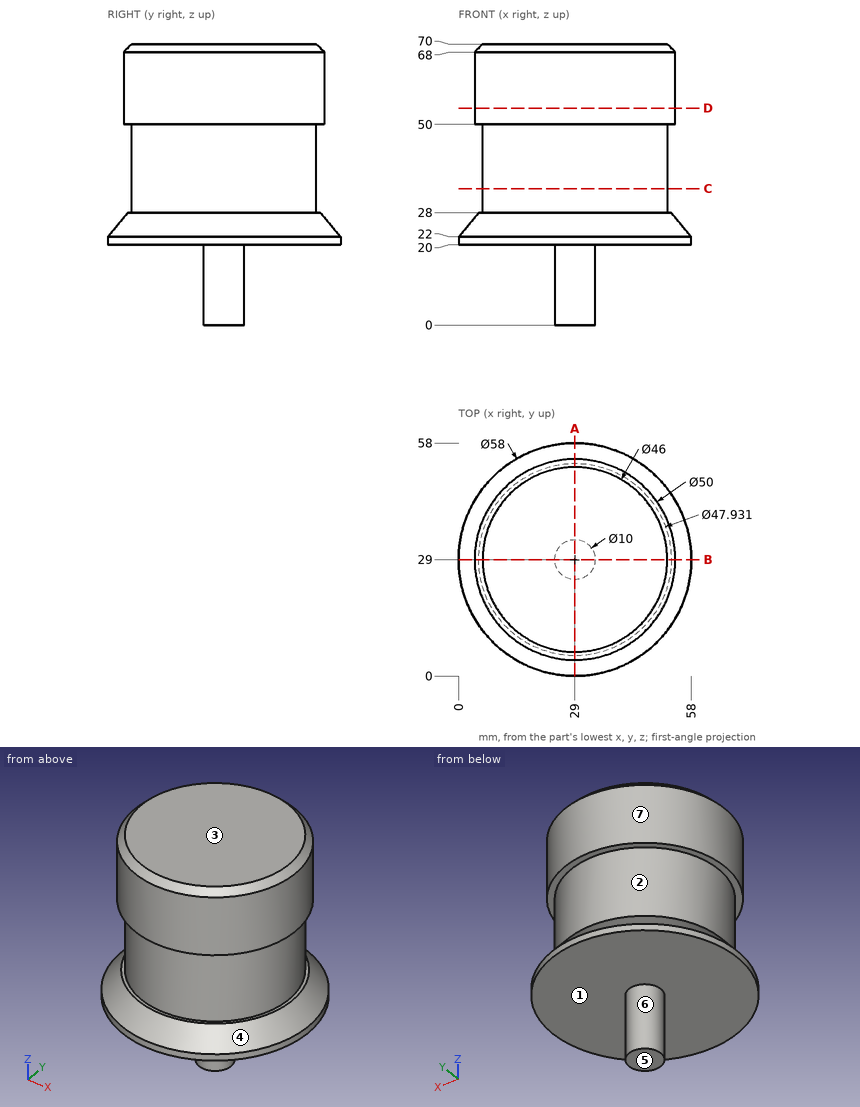
Drawing for the job (mm, zero at the part's lowest x, y, z). A direction names the side the tool comes from. Coordinates: 2 decimals unless noted, no trailing zeros. Order: outer loops, then holes, each group sorted by start corner. A loop starts at its lowest first (then second) coordinate and runs counter-clockwise, first axis right, second up. Notation, with made-up numbers: (83, 11.25) -> (92, 11.25) arc R13 ccw to (92, 17.25) -> close; hole circle Ø1 at (67, -27). An arc over 180 degrees is marked (long way). Return JSON: item names as keys, results as strings.
Item 1: Mould opens along Z. For the marked faces 1, 2, 3 and 4 say: pulls with the +Z half, pulls with the -Z half, needs draft (parallel to the pull), parting line crosses it, or undercut.
Model answer:
{"face 1": "pulls with the -Z half", "face 2": "undercut", "face 3": "pulls with the +Z half", "face 4": "undercut"}
Item 2: Slice it at A-A (x = 29). Write the cut outline in (y, z), then the cut area to 3 significant figures.
Model answer:
{"outline": "(0, 20) -> (24, 20) -> (24, 0) -> (34, 0) -> (34, 20) -> (58, 20) -> (58, 22) -> (52.97, 28) -> (52, 28) -> (52, 50) -> (54, 50) -> (54, 68) -> (52, 70) -> (6, 70) -> (4, 68) -> (4, 50) -> (6, 50) -> (6, 28) -> (5.03, 28) -> (0, 22) -> close", "area": "2,640 mm²"}
Item 3: 3-axis set-ups, long thin cutter, end or side, ignore diameter. For the marked faces 5, 6 and 7: which of +Z, -Z, +X, -X, +Y, -Y reach the whole face in a straight line?
Model answer:
{"face 5": "-Z, +X, -X, +Y, -Y", "face 6": "-Z", "face 7": "+Z"}
Item 4: Pin check, flat tips, straight feed: P1, Ø8, axis at y = 29.5, z = 14, coming from the -X side; P2, Ø6, axis at x = 28, z = 54.5, coming from the +Y side; P3, Ø6, axis at y = 24, z = 43.5, coming from the +X side. Stop position of each tip, or through.
Model answer:
{"P1": "stops at x = 24", "P2": "stops at y = 54", "P3": "stops at x = 51.91"}
Item 5: Slice it at D-D (z = 54). Write the cut outline in (x, y).
Model answer:
{"outline": "circle Ø50 at (29, 29)"}
Item 6: Wall check: line 1 along Y through (x, z) = (30, 30.5); line 2 along Z through (x, y) = (36.5, 36); line 3 along X through (y, z) = (41, 23.5). Give the ranges that are in metal, low to high. Write a range as from..to.
Model answer:
{"line 1": "y = 6.02..51.98", "line 2": "z = 20..70", "line 3": "x = 3.99..54.01"}
Item 7: Slice it at C-C (z = 34). Write the cut outline in (x, y).
Model answer:
{"outline": "circle Ø46 at (29, 29)"}
